Design review of the part shown in the three views and the two pictorial views. Dimensions are in mm from the part's minimum x, y and z. Round coordinates to 2 decimals unless told otherwise and drop trailing zeros. Loops run counter-clockwise (first coordinate to the right, second up) from the corner with the lowest first, then second, coordinate; pieces in that order, holes last. Notation, with made-up numbers: (-14, -12.75) -> (32, -12.75) arc R24 ccw to (32, 14.25) -> close; hole circle Ø9 at (32, -21). An arc over 180 degrees is marked (long way). Return JSON: item names as keys, results as strings. Group by question number.
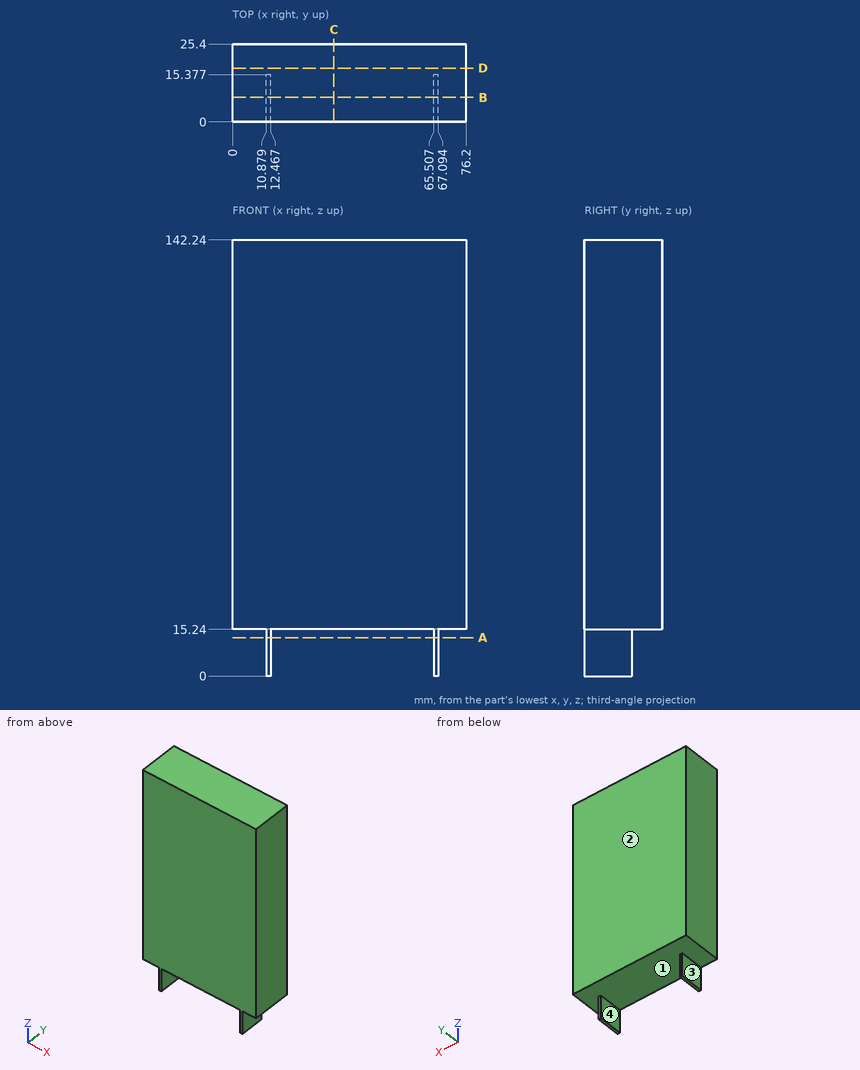
1. We need section A-A, the plane z = 12.5. Write out the cut boundary in (x, y) (1 decimal).
2. We need section B-B, the plane y = 8. Write out the cut boundary in (x, z) (1 decimal), then the cut area to 3 significant figures.
3. For P1, Ø7.5, axis at y = 4.5, z = 7, coming from the +X side; P2, Ø12, axis at x = 31, y = 11, coming from the -Z side; P3, Ø4.5, axis at y = 9, z = 5.5, coming from the -X side, all flat-tipped, find the tip position at first contact; note any pin that passes through.
4. We need section D-D, the plane y = 17.5. Write out the cut boundary in (x, z), then the cut area to 3 significant figures.
5. Draft analysis for pull direction X (two halves, no side actions). For the marked faces 1, 2, 3 and 4, state which applies: pulls with the +X half, pulls with the -X half, needs draft (parallel to the pull), parting line crosses it, or undercut.
6. We need section C-C, the plane x = 33. Write out the cut boundary in (y, z), then the cut area to 3 significant figures.
7. Wall thickness on line 1 (Z direction, x = 17, y = 11.5); line 2 (Y direction, x = 12, z = 11): over which ranges is each line inside the solid? List them lowest first.
Check sheet entries:
{
 "1": {"outline": "(10.9, 0) -> (12.5, 0) -> (12.5, 15.4) -> (10.9, 15.4) -> close; (65.5, 0) -> (67.1, 0) -> (67.1, 15.4) -> (65.5, 15.4) -> close"},
 "2": {"outline": "(0, 15.2) -> (10.9, 15.2) -> (10.9, 0) -> (12.5, 0) -> (12.5, 15.2) -> (65.5, 15.2) -> (65.5, 0) -> (67.1, 0) -> (67.1, 15.2) -> (76.2, 15.2) -> (76.2, 142.2) -> (0, 142.2) -> close", "area": "9,730 mm²"},
 "3": {"P1": "stops at x = 67.09", "P2": "stops at z = 15.24", "P3": "stops at x = 10.88"},
 "4": {"outline": "(0, 15.24) -> (76.2, 15.24) -> (76.2, 142.24) -> (0, 142.24) -> close", "area": "9,680 mm²"},
 "5": {"face 1": "undercut", "face 2": "needs draft", "face 3": "pulls with the -X half", "face 4": "undercut"},
 "6": {"outline": "(0, 15.24) -> (25.4, 15.24) -> (25.4, 142.24) -> (0, 142.24) -> close", "area": "3,230 mm²"},
 "7": {"line 1": "z = 15.24 to 142.24", "line 2": "y = 0 to 15.38"}
}
